Autodesk Inventor part; units mm, degrees
ref_plane "YZ Plane" through (0, 0, 0) normal (1, 0, 0) x (0, 1, 0)
ref_plane "XZ Plane" through (0, 0, 0) normal (0, 1, 0) x (-1, 0, 0)
ref_plane "XY Plane" through (0, 0, 0) normal (0, 0, 1) x (1, 0, 0)
sketch "Sketch1" plane through (0, 0, 0) normal (0, 0, 1) x (1, 0, 0)
  line L0 (-350, 95) -> (350, 95)
  line L1 (350, 95) -> (350, -95)
  line L2 (350, -95) -> (-350, -95)
  line L3 (-350, -95) -> (-350, 95)
  circle A0 centre (-250, 55) radius 10
  circle A1 centre (-250, -15) radius 10
  circle A2 centre (250, 55) radius 10
  circle A3 centre (250, -15) radius 10
  line L4 (-110, 95) -> (110, 95)
  point P0 (0, 0)
  point P1 (0, 95)
  point P2 (350, 0)
  point P3 (0, -155)
  dimension "d0" = 700
  dimension "d1" = 190
  dimension "d2" = 20
  dimension "d3" = 70
  dimension "d4" = 40
  dimension "d7" = 20
  dimension "d8" = 70
  dimension "d9" = 500
  dimension "d10" = 100
extrude "Extrusion1" add sketch "Sketch1" along normal blind 50
sketch "Sketch2" plane through (0, 0, 50) normal (0, 0, 1) x (1, 0, 0)
  line L0 (-110, 95) -> (110, 95)
  line L1 (110, 95) -> (110, -155)
  line L2 (110, -155) -> (-110, -155)
  line L3 (-110, -155) -> (-110, 95)
  line L4 (350, 95) -> (-350, 95)
  point P0 (0, 0)
  point P1 (0, -155)
  dimension "d15" = 220
  dimension "d16" = 250
extrude "Extrusion2" add sketch "Sketch2" along normal blind 30
sketch "Sketch3" plane through (0, 0, 50) normal (0, 0, -1) x (-1, 0, 0)
  line L0 (110, -95) -> (-110, -95)
  line L1 (-110, -95) -> (-110, -155)
  line L2 (-110, -155) -> (110, -155)
  line L3 (110, -155) -> (110, -95)
  point P0 (0, 0)
extrude "Extrusion3" add sketch "Sketch3" along normal blind 50
fillet "Fillet1" radius 50 4 edges at (-350, -95, 25) (-350, 95, 25) (350, -95, 25) (350, 95, 25)
scale "Scale1" factors (0.1, 0.1, 0.1) then translate (-225, -13.5, 0) bodies 1
equation "\"d7\" = d2"
equation "\"d10\" = -0.5 * d9 + 0.5 * d0"
properties part number "RotationLock"
Input: part model. Units: mm. Frame: model coordinates. A direction names the side the tool comes from. Coordinates: 2 decimals unless noted, no trailing zeros. Order: outer loops, then holes, each group sorted by start corner. A loop starts at its lowest first (then second) coordinate and runs counter-clockwise, first axis right, second up. Notation, with made-up numbers: M 34,46 L 43,46 A24 cw 43,70 Z; hole C -40,49 d4. An arc over 180 degrees is marked long. Answer in a Markdown table with one row per item.
(1) Draft query along X for faces 5 (the cylindrical face through (-250.8, -14.4, 2.5)), 6 (the flat face through (-225, -29, 4)), 7 (the cylindrical face through (-192, -22, 3)). Return one class per face: pulls with the +X half, pulls with the -X half, needs draft (parallel to the pull), parting line crosses it, or undercut.
Numbers:
| item | result |
|---|---|
| face 5 | undercut |
| face 6 | needs draft |
| face 7 | pulls with the +X half |
(2) Contact query for flat-ended pins moving along their axis: pin 1 Ø2 at (x, y) = (-214, -10.5) entering from -Z; pin 2 Ø9.5 at (x, y) = (-207, -15) entering from +Z; pin 3 Ø2.5 at (x, z) = (-202.5, 1.5) entering from -Y. Output: stop coordinate, or through.
Numbers:
| item | result |
|---|---|
| pin 1 | stops at z = 0 |
| pin 2 | stops at z = 5 |
| pin 3 | stops at y = -23 |
(3) Section query A-A, the plane x = -250. Output: boundary loops of the cut face in (y, z), plus the area to 3 significant figures.
Numbers:
| item | result |
|---|---|
| outline | M -23,0 L -16,0 L -16,5 L -23,5 Z; M -14,0 L -9,0 L -9,5 L -14,5 Z; M -7,0 L -4,0 L -4,5 L -7,5 Z |
| area | 75.0 mm^2 |
(4) Section query D-D, the plane y = -10.75. Output: boundary loops of the cut face in (x, z).
Numbers:
| item | result |
|---|---|
| outline | M -260,0 L -190,0 L -190,5 L -214,5 L -214,8 L -236,8 L -236,5 L -260,5 Z |
(5) Section query C-C, the plane z = 2. Output: boundary loops of the cut face in (x, y), plus the area to 3 significant figures.
Numbers:
| item | result |
|---|---|
| outline | M -260,-18 A5 ccw -255,-23 L -236,-23 L -236,-29 L -214,-29 L -214,-23 L -195,-23 A5 ccw -190,-18 L -190,-9 A5 ccw -195,-4 L -255,-4 A5 ccw -260,-9 Z; hole C -250,-15 d2; hole C -250,-8 d2; hole C -200,-15 d2; hole C -200,-8 d2 |
| area | 1,430 mm^2 |
(6) Section query B-B, the plane y = -15. Output: boundary loops of the cut face in (x, z).
Numbers:
| item | result |
|---|---|
| outline | M -260,0 L -251,0 L -251,5 L -260,5 Z; M -249,0 L -201,0 L -201,5 L -214,5 L -214,8 L -236,8 L -236,5 L -249,5 Z; M -199,0 L -190,0 L -190,5 L -199,5 Z |
(7) Material intervals for line 1 (Y direction, x = -250, z = 3.8); line 2 (Z direction, x = -246.5, y = -16); line 3 (Y direction, x = -254, z = 3.25), sorted ascending. Write a range as [from, to].
Numbers:
| item | result |
|---|---|
| line 1 | y = [-23, -16], [-14, -9], [-7, -4] |
| line 2 | z = [0, 5] |
| line 3 | y = [-23, -4] |
(8) Access query for faces 1 (the flat face through (-248, -13, 5)), 2 (the flat face through (-202, -13, 5)), 3 (the flat face through (-245, -23, 2)), 4 (the flat face through (-204, -23, 2)). Directions: +Z, -Z, +X, -X, +Y, -Y. A direction counts if a zero-diameter tool reaches every point of the face in a straight line with its end or side. Return the directions, or none.
Numbers:
| item | result |
|---|---|
| face 1 | +Z, -X, +Y, -Y |
| face 2 | +Z, +X, +Y, -Y |
| face 3 | +Z, -Z, -X, -Y |
| face 4 | +Z, -Z, +X, -Y |
